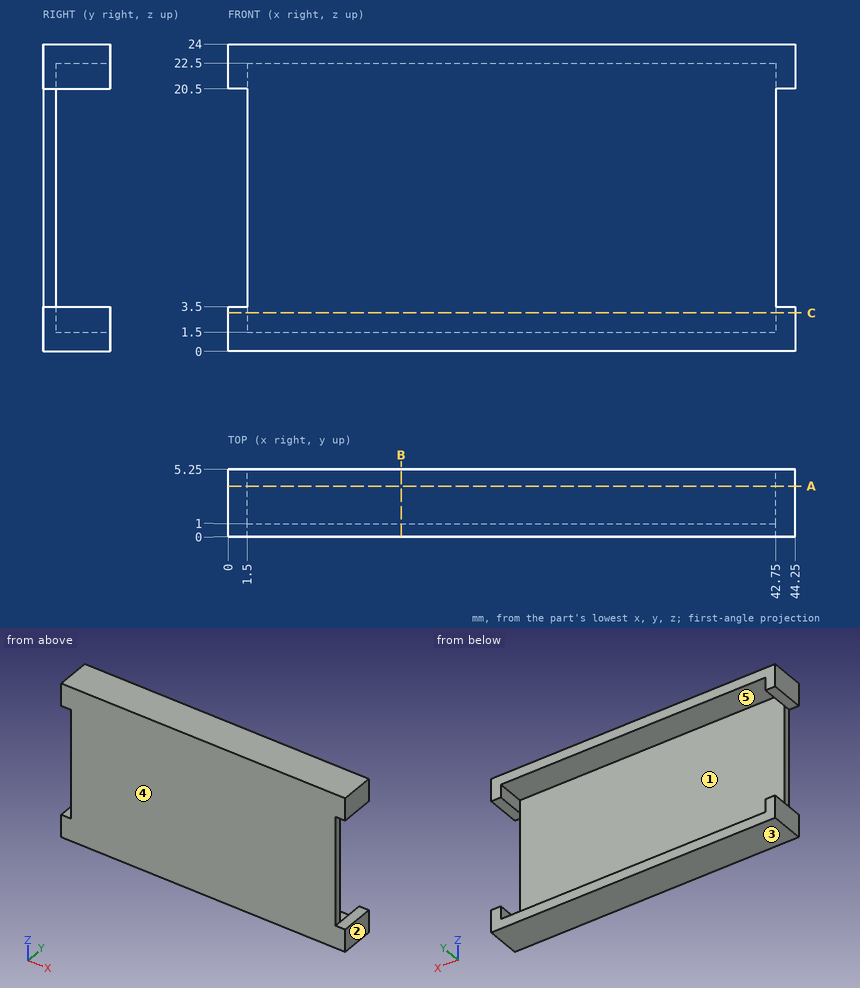
For this review, use the dimensioned drawing (mm, ordinates from the lowest corner) and the shaded views. A direction names the side the tool comes from. Coordinates: 2 decimals unless noted, no trailing zeros. Loops run counter-clockwise (first coordinate to the right, second up) from the corner with the lowest first, then second, coordinate; pieces in that order, holes last. Notation, with made-up numbers: (85.5, -21.75) -> (120.5, -21.75) arc R9 cw to (120.5, -17.75) -> close; hole circle Ø2 at (21, -28.5). An arc over 180 degrees is marked (long way). Return JSON: item names as keys, results as strings. Group by question number.
(1) Consider section C-C, the plane z = 3. Give the boundary of the cut face in (x, y), plus the area to 3 significant figures.
(2) For pin 1 Ø0.5 at (y, z) = (0.5, 13.5) entering from +X; pin 2 Ø5 at (x, z) = (39.5, 10.5) entering from +Y; pin 3 Ø0.5 at (y, z) = (0.5, 16) entering from -X, all flat-tipped, find the tip position at first contact; note any pin that passes through.
(3) To check wall thickness, follow L1, parallel to Z at x = 9, y = 2.75; L2, parallel to Y at x = 29.5, z = 16.5; L3, parallel to X at y = 0.6, z = 5.25. State the ranges of each line that lie inside material, in increasing order.
(4) Mouldability with a two-part tool opening along X and no side actions: class the marked faces 1, 2 and 3 as pulls with the +X half, pulls with the -X half, needs draft (parallel to the pull), parting line crosses it, or undercut.
(5) Tool access review of the marked faces 4 and 5: name each direction out of +Z, -Z, +X, -X, +Y, -Y from which nothing blocks a thin tool from reaching the whole face with its end or side.
(6) Consider section B-B, the plane x = 13.5. Give the boundary of the cut face in (y, z), plus the area to 4 significant figures.
(7) Consider section A-A, the plane y = 3.95. Give the boundary of the cut face in (x, z), plus the area to 3 significant figures.
Results below:
{
 "1": {"outline": "(0, 0) -> (44.25, 0) -> (44.25, 5.25) -> (42.75, 5.25) -> (42.75, 1) -> (1.5, 1) -> (1.5, 5.25) -> (0, 5.25) -> close", "area": "57.0 mm2"},
 "2": {"pin 1": "stops at x = 42.75", "pin 2": "stops at y = 1", "pin 3": "stops at x = 1.5"},
 "3": {"L1": "z = 0 to 1.5, 22.5 to 24", "L2": "y = 0 to 1", "L3": "x = 1.5 to 42.75"},
 "4": {"face 1": "undercut", "face 2": "pulls with the +X half", "face 3": "needs draft"},
 "5": {"face 4": "+Z, -Z, +X, -X, -Y", "face 5": "+Y"},
 "6": {"outline": "(0, 0) -> (5.25, 0) -> (5.25, 1.5) -> (1, 1.5) -> (1, 22.5) -> (5.25, 22.5) -> (5.25, 24) -> (0, 24) -> close", "area": "36.75 mm2"},
 "7": {"outline": "(0, 0) -> (44.25, 0) -> (44.25, 3.5) -> (42.75, 3.5) -> (42.75, 1.5) -> (1.5, 1.5) -> (1.5, 3.5) -> (0, 3.5) -> close; (0, 20.5) -> (1.5, 20.5) -> (1.5, 22.5) -> (42.75, 22.5) -> (42.75, 20.5) -> (44.25, 20.5) -> (44.25, 24) -> (0, 24) -> close", "area": "145 mm2"}
}
